Part model, mm, in its own coordinate system. Face numbers are marked on the shaded views. Coordinates: 2 decimals unless noted, no trailing zeros. Loops run counter-clockwise (first coordinate to the right, second up) from the corner with the lowest first, then second, coordinate; pieces in that order, holes last. Notation, with made-up numbers: (-37.5, -13.5) - (12.5, -13.5) arc R23 cw to (12.5, 10.5) - close; hole circle Ø4 at (-30, -32.5). An arc over 180 degrees is marked (long way). Use a Markdown table: item, result. Add a question column.
1. Drop flat-ended pins along their axis: pin 1 (16.5 mm diameter, centred on x = 34.5, z = -6, fed in from +Y); pin 2 (2 mm diameter, centred on x = 26, z = 13, fed in from -Y); pin 3 (6 mm diameter, centred on y = 3, z = -26.5, fed in from +X); pin 4 (10 mm diameter, centred on x = 60, z = -6.5, fed in from +Y). Give the stop position or say it passes through.
2. Wall check: probe 1 along X at (y, z) = (30.4, 0); probe 2 along Z at (x, y) = (64.5, -19.5); probe 3 along Z at (x, y) = (12, -19). Give the ranges that are in metal, low to high. Write a range as [from, to].
3. Band-saw the part on B-B, the plane x = 65. Give the cut face in (y, z), plus the area to 3 significant figures.
4. Band-saw the part on C-C, the plane z = 26.5. Give the cut face in (x, y).
5. Band-saw the part on D-D, the plane y = 19.5. Give the cut face in (x, z), plus the area to 3 significant figures.
6. Pull direction Z, two halves, no side cores. Call the marked faces 1 and 2: pulls with the +Z half, pulls with the -Z half, needs draft (parallel to the pull), parting line crosses it, or undercut.
7. Band-saw the part on A-A, the plane y = -14. Give the cut face in (x, z).
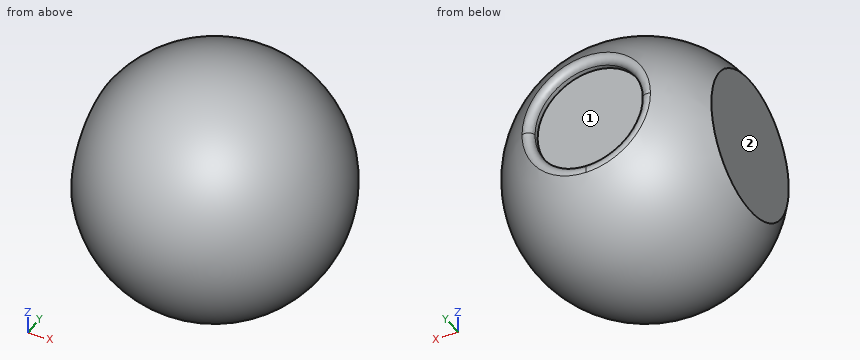
from build123d import *

# Parameters (mm, degrees)
KES_EKSTR_ZYON1_DEPTH      = 95.305355097
KES_EKSTR_ZYON1_DEPTH_BACK = 95.305355097
IZIM3_W                    = 6.7
IZIM3_H                    = 83.072589547
KES_EKSTR_ZYON2_START      = 30
IZIM4_R                    = 16.5
KES_EKSTR_ZYON2_DEPTH      = 65.305355097
RADYUS1_R                  = 2


with BuildPart() as part:
    # Çizim2 → Döndür1 (revolve)
    with BuildSketch(Plane.XY):
        with BuildLine():
            Line((77, 0), (0, 0))
            ThreePointArc((0, 0), (38.5, 38.5), (77, 0))
        make_face()
    revolve(axis=Axis((77, 0, 0), (-1, 0, 0)))

    # Çizim3 → Kes-Ekstrüzyon1 (cut, two sides: drawn at the far end of the back side and taken through both)
    with BuildSketch(Plane(origin=(0, 0, 0), x_dir=(1, 0, 0), z_dir=(0, 1, 0)).offset(-KES_EKSTR_ZYON1_DEPTH_BACK)):
        with Locations((3.35, -0.927609561)):
            Rectangle(IZIM3_W, IZIM3_H)
    extrude(amount=KES_EKSTR_ZYON1_DEPTH + KES_EKSTR_ZYON1_DEPTH_BACK, mode=Mode.SUBTRACT)

    # Çizim4 → Kes-Ekstrüzyon2 (cut, through all)
    with BuildSketch(Plane(origin=(0, 0, 0), x_dir=(1, 0, 0), z_dir=(0, 1, 0)).offset(KES_EKSTR_ZYON2_START)):
        with Locations(Location((38.5, 0, 0), (0, 0, 90))):
            Circle(IZIM4_R)
    extrude(amount=KES_EKSTR_ZYON2_DEPTH, mode=Mode.SUBTRACT)

    # Radyus1
    radyus1_edges = [part.edges().sort_by_distance(p)[0] for p in [
        (26.832738111, 34.785054262, -11.667261889),
    ]]
    fillet(radyus1_edges, radius=RADYUS1_R)


solid = part.part
Geometry check:
| question | item | result |
|---|---|---|
| 1 | pin 1 | stops at y = 30 |
| 1 | pin 2 | stops at y = -34.53 |
| 1 | pin 3 | stops at x = 68.86 |
| 1 | pin 4 | stops at y = 33.46 |
| 2 | probe 1 | x = [14.88, 22], [55, 62.12] |
| 2 | probe 2 | z = [-20.64, 20.64] |
| 2 | probe 3 | z = [-20.47, 20.47] |
| 3 | outline | circle Ø55.86 at (0, 0) |
| 3 | area | 2,450 mm^2 |
| 4 | outline | circle Ø55.86 at (38.5, 0) |
| 5 | outline | (6.7, -9.53) arc R33.2 ccw (long way) to (6.7, 9.53) - close |
| 5 | area | 3,440 mm^2 |
| 6 | face 1 | undercut |
| 6 | face 2 | needs draft |
| 7 | outline | (6.7, -16.58) arc R35.86 ccw (long way) to (6.7, 16.58) - close |
